```python
from build123d import *

# Parameters (mm, degrees)
SKETCH1_R           = 3.75
BOSS_EXTRUDE1_DEPTH = 5
SKETCH2_R           = 5
BOSS_EXTRUDE2_DEPTH = 2
BOSS_EXTRUDE3_DEPTH = 11.4
SKETCH4_R           = 3.204293994
BOSS_EXTRUDE4_DEPTH = 7
BOSS_EXTRUDE5_DEPTH = 10


with BuildPart() as part:
    # Sketch1 → Boss-Extrude1 (new body)
    with BuildSketch(Plane.XY):
        Circle(SKETCH1_R)
    extrude(amount=BOSS_EXTRUDE1_DEPTH)

    # Sketch2 → Boss-Extrude2 (add)
    with BuildSketch(Plane.XY.offset(5)):
        Circle(SKETCH2_R)
    extrude(amount=BOSS_EXTRUDE2_DEPTH)

    # Sketch3 → Boss-Extrude3 (add)
    with BuildSketch(Plane.XY.offset(7)):
        Polygon((3.7, 0), (1.85, 3.204293994), (-1.85, 3.204293994), (-3.7, 0), (-1.85, -3.204293994), (1.85, -3.204293994), align=None)
    extrude(amount=BOSS_EXTRUDE3_DEPTH)

    # Sketch4 → Boss-Extrude4 (add)
    with BuildSketch(Plane.XY.offset(18.4)):
        Circle(SKETCH4_R)
    extrude(amount=BOSS_EXTRUDE4_DEPTH)

    # Sketch5 → Boss-Extrude5 (add)
    with BuildSketch(Plane.XY.offset(25.4)):
        Polygon((3.175, 0), (1.5875, 2.749630657), (-1.5875, 2.749630657), (-3.175, 0), (-1.5875, -2.749630657), (1.5875, -2.749630657), align=None)
    extrude(amount=BOSS_EXTRUDE5_DEPTH)


solid = part.part
```
Check sheet for the modelled part. Datum: model origin and axes. Units: mm. A direction names the side the tool comes from. Round coordinates to 2 decimals unless told otherwise and drop trailing zeros. Loops run counter-clockwise (first coordinate to the right, second up) from the corner with the lowest first, then second, coordinate; pieces in that order, holes last. Notation, with made-up numbers: M -39.5,40 L -4.5,40 A29 cw -4.5,63 Z; hole C 50.5,-40 d8. An arc over 180 degrees is marked long. Answer as a JSON object with one key per item and string values.
1. Section check D-D (x = 4.25). Record the boundary of the cut face in (y, z).
Reply:
{"outline": "M -2.63,5 L 2.63,5 L 2.63,7 L -2.63,7 Z"}
2. Section check A-A (z = 15.5). Record the boundary of the cut face in (x, y).
Reply:
{"outline": "M -3.7,0 L -1.85,-3.2 L 1.85,-3.2 L 3.7,0 L 1.85,3.2 L -1.85,3.2 Z"}
3. Section check C-C (x = 2.25). Record the boundary of the cut face in (y, z), plus the area to 3 significant figures.
Reply:
{"outline": "M -4.47,5 L -3,5 L -3,0 L 3,0 L 3,5 L 4.47,5 L 4.47,7 L 2.51,7 L 2.51,18.4 L 2.28,18.4 L 2.28,25.4 L 1.6,25.4 L 1.6,35.4 L -1.6,35.4 L -1.6,25.4 L -2.28,25.4 L -2.28,18.4 L -2.51,18.4 L -2.51,7 L -4.47,7 Z", "area": "169 mm²"}
4. Gauge pin test, flat ends, axial feed: P1, Ø1, axis at y = -2, z = 19, coming from the -X side; P2, Ø4, axis at x = -3, z = 14, coming from the -Y side; P3, Ø2.5, axis at x = -0.5, z = 31, coming from the +Y side. Record the tip position at first contact, or that the pin passes through.
Reply:
{"P1": "stops at x = -2.83", "P2": "stops at y = -3.2", "P3": "stops at y = 2.75"}
5. Scan lines: line 1 (Z direction, x = -0.25, y = 3); line 2 (Z direction, x = 1.5, y = -3.5); line 3 (X direction, y = -0.25, z = 5.5). Record each from-to range of solid material in increasing order.
Reply:
{"line 1": "z = 0 to 25.4", "line 2": "z = 5 to 7", "line 3": "x = -4.99 to 4.99"}
6. Access from +Z, -Z, +X, -X, +Y, -Y to the whole of each face (thin tool, end or side, straight path). Record for faces 1 (the flat face through (0, -2.75, 30)), 2 (the flat face through (2.39, 1.36, 30.33)), 3 (the flat face through (0, 3.204, 13)).
Reply:
{"face 1": "+Z, +X, -X, -Y", "face 2": "+Z, +X, +Y", "face 3": "+Z, +X, -X, +Y"}
7. Section check B-B (x = -1). Record the boundary of the cut face in (y, z).
Reply:
{"outline": "M -4.9,5 L -3.61,5 L -3.61,0 L 3.61,0 L 3.61,5 L 4.9,5 L 4.9,7 L 3.2,7 L 3.2,18.4 L 3.04,18.4 L 3.04,25.4 L 2.75,25.4 L 2.75,35.4 L -2.75,35.4 L -2.75,25.4 L -3.04,25.4 L -3.04,18.4 L -3.2,18.4 L -3.2,7 L -4.9,7 Z"}
